Could you check a few things on this model? Use its own coordinates, in mm. A direction names the side the tool comes from. Coordinates: 2 decimals unless noted, no trailing zeros. Order: outer loops, then holes, each group sorted by start corner. A loop starts at its lowest first (then second) coordinate and runs counter-clockwise, first axis right, second up. Notation, with made-up numbers: M -35,-18.75 L 16,-18.75 A13 ccw 16,-1.75 Z; hole C 2.25,-32.75 d3. An arc over 180 degrees is marked long. Write item = value, one per line. Start each with the question number.
from build123d import *

# Parameters (mm, degrees)
SKETCH_W        = 85
SKETCH_H        = 25
PAD_DEPTH       = 17
SKETCH001_W     = 81
SKETCH001_H     = 21
POCKET_DEPTH    = 15
SKETCH002_W     = 16
SKETCH002_H     = 12
POCKET001_DEPTH = 8
SKETCH003_W     = 83
SKETCH003_H     = 23
POCKET002_DEPTH = 2
SKETCH004_W     = 5
SKETCH004_H     = 5
PAD001_DEPTH    = 2.5
SKETCH008_W     = 12
SKETCH008_H     = 25
PAD004_DEPTH    = 4
SKETCH010_W     = 12
SKETCH010_H     = 25
PAD005_DEPTH    = 4
SKETCH011_R     = 2.5
POCKET004_DEPTH = 4.001
SKETCH012_R     = 2.5
POCKET005_DEPTH = 4.001


with BuildPart() as part:
    # Sketch → Pad (new body)
    with BuildSketch(Plane.XY):
        with Locations((42.5, 12.5)):
            Rectangle(SKETCH_W, SKETCH_H)
    extrude(amount=PAD_DEPTH)

    # Sketch001 (on Face6 of Pad) → Pocket (cut)
    with BuildSketch(Plane.XY.offset(17)):
        with Locations((42.5, 12.5)):
            Rectangle(SKETCH001_W, SKETCH001_H)
    extrude(amount=-POCKET_DEPTH, mode=Mode.SUBTRACT)

    # Sketch002 → Pocket001 (cut)
    with BuildSketch(Plane.XY):
        with Locations((57.5, 6)):
            Rectangle(SKETCH002_W, SKETCH002_H)
    extrude(amount=POCKET001_DEPTH, mode=Mode.SUBTRACT)

    # Sketch003 (on Face7 of Pocket001) → Pocket002 (cut)
    with BuildSketch(Plane.XY.offset(17)):
        with Locations((42.5, 12.5)):
            Rectangle(SKETCH003_W, SKETCH003_H)
    extrude(amount=-POCKET002_DEPTH, mode=Mode.SUBTRACT)

    # Sketch004 (on Face12 of Pocket002) → Pad001 (join)
    with BuildSketch(Plane.XY.offset(2)):
        with Locations((2.5, 2.5)):
            Rectangle(SKETCH004_W, SKETCH004_H)
        with Locations((2.5, 22.5)):
            Rectangle(SKETCH004_W, SKETCH004_H)
        with Locations((82.5, 2.5)):
            Rectangle(SKETCH004_W, SKETCH004_H)
        with Locations((82.5, 22.5)):
            Rectangle(SKETCH004_W, SKETCH004_H)
    extrude(amount=PAD001_DEPTH)

    # Sketch008 → Pad004 (join)
    with BuildSketch(Plane.XY):
        with Locations((-6, 12.5)):
            Rectangle(SKETCH008_W, SKETCH008_H)
    extrude(amount=PAD004_DEPTH)

    # Sketch010 → Pad005 (join)
    with BuildSketch(Plane.XY):
        with Locations((91, 12.5)):
            Rectangle(SKETCH010_W, SKETCH010_H)
    extrude(amount=PAD005_DEPTH)

    # Sketch011 (on Face27 of Pad005) → Pocket004 (cut, through all)
    with BuildSketch(Plane.XY.offset(4)):
        with Locations((-6, 12.5)):
            Circle(SKETCH011_R)
    extrude(amount=-POCKET004_DEPTH, mode=Mode.SUBTRACT)

    # Sketch012 (on Face20 of Pocket004) → Pocket005 (cut, through all)
    with BuildSketch(Plane.XY.offset(4)):
        with Locations((91, 12.5)):
            Circle(SKETCH012_R)
    extrude(amount=-POCKET005_DEPTH, mode=Mode.SUBTRACT)


solid = part.part
(1) Imagine slicing it at A-A on x = -6. List the corners of the cut face in (y, z) for me.
(2) Will these pins go through, and if not, where does the flat tip stop? P1, Ø3.5, axis at x = 93, y = 13, coming from the +Z side; P2, Ø5, axis at y = 3.5, z = 7.5, coming from the +X side; P3, Ø10, axis at y = 14.5, z = 10.5, coming from the -X side.
(3) Imagine slicing it at B-B on z = 1. List the corners of the cut face in (x, y) for me, plus the area to 3 significant figures.
(4) For faces 4 (the flat face through (0, 12, 10)), 5 (the flat face through (65.5, 3, 1)), 6 (the flat face through (5, 3, 3)), which set-ups out of +Z, -Z, +X, -X, +Y, -Y let a thin tool reach every point of the face, with its end or its side?
(5) Please list where these lines run through material, in increasing order: probe 1 along Y at (x, z) = (91, 1.55); probe 2 along Y at (x, z) = (15, 5); probe 3 along X at (y, z) = (21.5, 11.25). Write a range as from..to.
(6) Thinking about a two-plate mould opening in Y: for faces 1 (the flat face through (42, 0, 8)), 2 (the flat face through (42.3, 0.5, 17)), 3 (the cylindrical face through (-4.85, 10.28, 2.03)), which applies, released by +Y, released by -Y, zero draft, split by the parting line, or undercut?
(7) Imagine slicing it at D-D on z = 11. List the corners of the cut face in (x, y) for me, plus the area to 3 significant figures.
(8) Imagine slicing it at C-C on y = 7.5. List the corners of the cut face in (x, z) for me, plus the area to 3 significant figures.
Response:
q1.outline = M 0,0 L 10,0 L 10,4 L 0,4 Z; M 15,0 L 25,0 L 25,4 L 15,4 Z
q2.P1 = 4
q2.P2 = 85
q2.P3 = 0
q3.outline = M -12,0 L 49.5,0 L 49.5,12 L 65.5,12 L 65.5,0 L 97,0 L 97,25 L -12,25 Z; hole C -6,12.5 d5; hole C 91,12.5 d5
q3.area = 2,490 mm2
q4.face_4 = +Z, -X, +Y, -Y
q4.face_5 = -Z, -Y
q4.face_6 = +Z
q5.probe_1 = 0..10, 15..25
q5.probe_2 = 0..2, 23..25
q5.probe_3 = 0..2, 83..85
q6.face_1 = released by -Y
q6.face_2 = zero draft
q6.face_3 = undercut
q7.outline = M 0,0 L 85,0 L 85,25 L 0,25 Z; hole M 2,2 L 83,2 L 83,23 L 2,23 Z
q7.area = 424 mm2
q8.outline = M -12,0 L 49.5,0 L 49.5,2 L 2,2 L 2,15 L 1,15 L 1,17 L 0,17 L 0,4 L -12,4 Z; M 65.5,0 L 97,0 L 97,4 L 85,4 L 85,17 L 84,17 L 84,15 L 83,15 L 83,2 L 65.5,2 Z
q8.area = 290 mm2
